Build history of the part. All positions in model axes, mm. A direction names the side the tool comes from. Round coordinates to 2 decimals unless told otherwise and drop trailing zeros. Write each loop counter-clockwise with the first axis right and the second up, starting at its lowest first coordinate (ties: lowest second). Pieces come first, ordered by that corner, then holes.
Item 1: Band-saw the part on C-C, the plane z = 4.75. Count the separate pieces of the cut face and the enclosed holes in it, then the cut area to 3 significant figures.
Item 2: Band-saw the part on D-D, the plane x = 9. Write the cut outline in (y, z).
Item 3: Mould opens along Z. For faces 4 (the cylindrical face through (14.707, -7.337, 4.596)), 5 (the flat face through (12, -4, 0)), 6 (the flat face through (8.97, -7.83, 5.35)) say: +Z half, -Z half, draft (parallel to the pull), parting line (faces both ways), or undercut.
Item 4: Band-saw the part on A-A, the plane y = -2.5. Write the cut outline in (x, z) (3 decimals), then the cut area to 3 significant figures.
Item 5: Band-saw the part on B-B, the plane x = 1.75. Write the cut outline in (y, z).
Item 6: Wall check: probe 1 along X at (y, z) = (-3.25, 5.75); probe 2 along X at (y, z) = (-4.25, 5); probe 3 along Y at (x, z) = (3.75, 6.25). Give the ranges that are in metal, low to high.
Item 7: 3-axis set-ups, long thin cutter, end or side, ignore diameter. For faces 1 (the cylindrical face through (21.92, -3.87, 4.4)), 2 (the flat face through (22, -6.83, 5)), 3 (the flat face through (22, -1, 5)): which of +Z, -Z, +X, -X, +Y, -Y reach the whole face in a straight line?
Item 8: Drop flat-ended pins along their axis: pin 1 Ø3 at (x, z) = (3.5, 5) entering from -Y; pin 2 Ø1 at (y, z) = (-3.5, 2.5) entering from +X. Give the stop position or say it passes through.
```python
from build123d import *

# Parameters (mm, degrees)
F0_R     = 2.45
F1_DEPTH = 7.83
F2_DEPTH = 1
F3_R     = 3.1
F3_R_2   = 2.45
F4_DEPTH = 1


with BuildPart() as f1:
    # F0 (on Front) → F1 (new body)
    with BuildSketch(Plane.XZ):
        with BuildLine():
            ThreePointArc((0, 3.665), (1.073454, 1.073454), (3.665, 0))
            Line((3.665, 0), (19.835, 0))
            ThreePointArc((19.835, 0), (22.426546, 1.073454), (23.5, 3.665))
            ThreePointArc((23.5, 3.665), (22.426546, 6.256546), (19.835, 7.33))
            Line((19.835, 7.33), (15.666667, 7.33))
            Line((15.666667, 7.33), (7.833667, 7.33))
            Line((7.833667, 7.33), (3.665, 7.33))
            ThreePointArc((3.665, 7.33), (1.073454, 6.256546), (0, 3.665))
        make_face()
        with BuildLine():
            ThreePointArc((10.166571, 1), (8.650167, 3.665), (10.166571, 6.33))
            ThreePointArc((10.166571, 6.33), (11.750167, 6.765), (13.333762, 6.33))
            ThreePointArc((13.333762, 6.33), (14.850167, 3.665), (13.333762, 1))
            ThreePointArc((13.333762, 1), (11.750167, 0.565), (10.166571, 1))
        make_face(mode=Mode.SUBTRACT)
        with BuildLine():
            ThreePointArc((17.999738, 1), (16.483333, 3.665), (17.999738, 6.33))
            ThreePointArc((17.999738, 6.33), (22.683333, 3.665), (17.999738, 1))
        make_face(mode=Mode.SUBTRACT)
        with BuildLine():
            ThreePointArc((5.500429, 1), (0.816833, 3.665), (5.500429, 6.33))
            ThreePointArc((5.500429, 6.33), (7.016833, 3.665), (5.500429, 1))
        make_face(mode=Mode.SUBTRACT)
        with BuildLine():
            ThreePointArc((5.500429, 1), (7.016833, 3.665), (5.500429, 6.33))
            ThreePointArc((5.500429, 6.33), (0.816833, 3.665), (5.500429, 1))
        make_face()
        with Locations((3.916833, 3.665)):
            Circle(F0_R, mode=Mode.SUBTRACT)
        with BuildLine():
            ThreePointArc((13.333762, 6.33), (11.750167, 6.765), (10.166571, 6.33))
            ThreePointArc((10.166571, 6.33), (8.650167, 3.665), (10.166571, 1))
            ThreePointArc((10.166571, 1), (11.750167, 0.565), (13.333762, 1))
            ThreePointArc((13.333762, 1), (14.850167, 3.665), (13.333762, 6.33))
        make_face()
        with Locations((11.750167, 3.665)):
            Circle(F0_R, mode=Mode.SUBTRACT)
        with BuildLine():
            ThreePointArc((17.999738, 1), (22.683333, 3.665), (17.999738, 6.33))
            ThreePointArc((17.999738, 6.33), (16.483333, 3.665), (17.999738, 1))
        make_face()
        with Locations((19.583333, 3.665)):
            Circle(F0_R, mode=Mode.SUBTRACT)
    extrude(amount=F1_DEPTH)

    # F0 (on Front) → F2 (cut)
    with BuildSketch(Plane.XZ):
        with BuildLine():
            ThreePointArc((5.500429, 1), (7.016833, 3.665), (5.500429, 6.33))
            ThreePointArc((5.500429, 6.33), (0.816833, 3.665), (5.500429, 1))
        make_face()
        with Locations((3.916833, 3.665)):
            Circle(F0_R, mode=Mode.SUBTRACT)
        with BuildLine():
            ThreePointArc((13.333762, 6.33), (11.750167, 6.765), (10.166571, 6.33))
            ThreePointArc((10.166571, 6.33), (8.650167, 3.665), (10.166571, 1))
            ThreePointArc((10.166571, 1), (11.750167, 0.565), (13.333762, 1))
            ThreePointArc((13.333762, 1), (14.850167, 3.665), (13.333762, 6.33))
        make_face()
        with Locations((11.750167, 3.665)):
            Circle(F0_R, mode=Mode.SUBTRACT)
        with BuildLine():
            ThreePointArc((17.999738, 1), (22.683333, 3.665), (17.999738, 6.33))
            ThreePointArc((17.999738, 6.33), (16.483333, 3.665), (17.999738, 1))
        make_face()
        with Locations((19.583333, 3.665)):
            Circle(F0_R, mode=Mode.SUBTRACT)
    extrude(amount=F2_DEPTH, mode=Mode.SUBTRACT)

    # F3 (on face) → F4 (cut)
    with BuildSketch(Plane.XZ.offset(7.83)):
        with Locations((3.916833, 3.665)):
            Circle(F3_R)
        with Locations((3.916833, 3.665)):
            Circle(F3_R_2, mode=Mode.SUBTRACT)
        with Locations((11.750167, 3.665)):
            Circle(F3_R)
        with Locations((11.750167, 3.665)):
            Circle(F3_R_2, mode=Mode.SUBTRACT)
        with Locations((19.583333, 3.665)):
            Circle(F3_R)
        with Locations((19.583333, 3.665)):
            Circle(F3_R_2, mode=Mode.SUBTRACT)
    extrude(amount=-F4_DEPTH, mode=Mode.SUBTRACT)


solid = f1.part
```
Results:
1. separate pieces: 4
1. enclosed holes: 0
1. area: 69.7 mm2
2. outline: (-7.83, 0) - (0, 0) - (0, 2.23) - (-1, 2.23) - (-1, 5.1) - (0, 5.1) - (0, 7.33) - (-7.83, 7.33) - (-7.83, 5.1) - (-6.83, 5.1) - (-6.83, 2.23) - (-7.83, 2.23) - close
3. face 4: undercut
3. face 5: -Z half
3. face 6: draft
4. outline: (0, 3.665) arc R3.665 ccw to (3.665, 0) - (19.835, 0) arc R3.665 ccw to (23.5, 3.665) arc R3.665 ccw to (19.835, 7.33) - (3.665, 7.33) arc R3.665 ccw to start; hole circle Ø4.9 at (3.917, 3.665); hole circle Ø4.9 at (11.75, 3.665); hole circle Ø4.9 at (19.583, 3.665)
4. area: 104 mm2
5. outline: (-7.83, 0.54) - (0, 0.54) - (0, 1.45) - (-1, 1.45) - (-1, 2.52) - (-6.83, 2.52) - (-6.83, 1.45) - (-7.83, 1.45) - close; (-7.83, 5.88) - (-6.83, 5.88) - (-6.83, 4.81) - (-1, 4.81) - (-1, 5.88) - (0, 5.88) - (0, 6.79) - (-7.83, 6.79) - close
6. probe 1: x = 0.65 to 2.63, 5.2 to 10.46, 13.04 to 18.3, 20.87 to 22.85
6. probe 2: x = 0.25 to 1.86, 5.97 to 9.7, 13.8 to 17.53, 21.64 to 23.25
6. probe 3: y = -6.83 to -1
7. face 1: +Y, -Y
7. face 2: -Y
7. face 3: +Y
8. pin 1: stops at y = -6.83
8. pin 2: stops at x = 23.44
